Source: CAD feature listing. Evaluate the final solid. Frame: model axes, mm. A direction names the side the tool comes from. Give positions to 0.01 mm unless a question says otherwise; leave off trailing zeros. Loops run counter-clockwise (first coordinate to the right, second up) from the corner with the lowest first, then second, coordinate; pieces in that order, holes last. Notation, with made-up numbers: (-39, -28.5) -> (-8, -28.5) arc R11 cw to (-8, -10.5) -> close; hole circle Ø3 at (53.5, 29.25). An arc over 180 degrees is marked (long way). Return JSON: item names as keys, results as strings. Group by question number.
```python
from build123d import *

# Parameters (mm, degrees)
BOSS_EXTRUDE1_DEPTH = 1.3
SKETCH2_W           = 1.4
SKETCH2_H           = 18
BOSS_EXTRUDE2_DEPTH = 1.3
SKETCH2_3_W         = 25
SKETCH2_3_H         = 16
CUT_EXTRUDE1_DEPTH  = 55.166871794
CUT_EXTRUDE2_DEPTH  = 55.166871794
SKETCH7_W           = 1
SKETCH7_H           = 14
CUT_EXTRUDE3_DEPTH  = 55.166871794


with BuildPart() as part:
    # Sketch1 → Boss-Extrude1 (new body)
    with BuildSketch(Plane(origin=(0, 0, 0), x_dir=(1, 0, 0), z_dir=(0, 1, 0))):
        Polygon((-43, 31), (43, 31), (43, -20), (32, -31), (-32, -31), (-43, -20), align=None)
    extrude(amount=BOSS_EXTRUDE1_DEPTH)

    # Sketch2 → Boss-Extrude2 (add)
    with BuildSketch(Plane(origin=(0, 0, 0), x_dir=(1, 0, 0), z_dir=(0, 1, 0))):
        with Locations((43.7, 2)):
            Rectangle(SKETCH2_W, SKETCH2_H)
        with Locations((-43.7, 2)):
            Rectangle(SKETCH2_W, SKETCH2_H)
    extrude(amount=BOSS_EXTRUDE2_DEPTH)

    # Sketch2<3> → Cut-Extrude1 (cut, through all)
    with BuildSketch(Plane(origin=(0, 0, 0), x_dir=(1, 0, 0), z_dir=(0, 1, 0))):
        with Locations((0, 23)):
            Rectangle(SKETCH2_3_W, SKETCH2_3_H)
    extrude(amount=CUT_EXTRUDE1_DEPTH, mode=Mode.SUBTRACT)

    # Sketch6 → Cut-Extrude2 (cut, through all)
    with BuildSketch(Plane(origin=(0, 1.3, 0), x_dir=(1, 0, 0), z_dir=(0, 1, 0))):
        with BuildLine():
            Line((-43, 31), (43, 31))
            ThreePointArc((43, 31), (0, 23.231359566), (-43, 31))
        make_face()
    extrude(amount=-CUT_EXTRUDE2_DEPTH, mode=Mode.SUBTRACT)

    # Sketch7 → Cut-Extrude3 (cut, through all)
    with BuildSketch(Plane(origin=(0, 1.3, 0), x_dir=(1, 0, 0), z_dir=(0, 1, 0))):
        with Locations((-10.5, -5.25)):
            Rectangle(SKETCH7_W, SKETCH7_H)
        with Locations((10.5, -5.25)):
            Rectangle(SKETCH7_W, SKETCH7_H)
    extrude(amount=-CUT_EXTRUDE3_DEPTH, mode=Mode.SUBTRACT)


solid = part.part
```
1) Reachability of faces 1 (the face through (1, 1.3, 0)), 2 (the face through (-27.764, 0.659, -26.409)) from +Z, -Z, +X, -X, +Y, -Y: full face, straight path, thin tool, end or side. Return the list, or none.
2) Mould query, pull axis X, two halves, no side actions, for faces 3 (the face through (28.19, 0.66, -26.51)), 4 (the face through (1, 0, 0)), 5 (the face through (38, 1, 25)). Classes: released by +X, released by -X, zero draft, split by the parting line, or undercut.
3) Material intervals for line 1 (X direction, y = 0.5, z = 8.5); line 2 (X direction, y = 0.6, z = 3); line 3 (X direction, y = 0.1, z = 17.5), sorted ascending.
4) Cut plane C-C on z = -21. Return loops of the section in (x, y).
5) Cut plane A-A on z = 8. Return loops of the section in (x, y).
6) Contact query for flat-ended pins moving along their axis: P1, Ø0.6, axis at x = 44, y = 1, coming from the -Z side; P2, Ø0.6, axis at y = 0.5, z = -18.5, coming from the -X side; P3, Ø0.6, axis at y = 1, z = -20.5, coming from the +X side. Output: stop coordinate, or through.
7) Cut plane B-B on y = 1.05. Return loops of the section in (x, z), then the cut area to 3 significant figures.
8) Cut plane D-D on x = -2. Return loops of the section in (y, z).
Calculated:
{
 "1": {"face 1": "+Z, -Z, +X, -X, +Y", "face 2": "-Z, +Y, -Y"},
 "2": {"face 3": "undercut", "face 4": "zero draft", "face 5": "released by +X"},
 "3": {"line 1": "-43 to -11, -10 to 10, 11 to 43", "line 2": "-44.4 to -11, -10 to 10, 11 to 44.4", "line 3": "-43 to 43"},
 "4": {"outline": "(-43, 0) -> (-12.5, 0) -> (-12.5, 1.3) -> (-43, 1.3) -> close; (12.5, 0) -> (43, 0) -> (43, 1.3) -> (12.5, 1.3) -> close"},
 "5": {"outline": "(-43, 0) -> (-11, 0) -> (-11, 1.3) -> (-43, 1.3) -> close; (-10, 0) -> (10, 0) -> (10, 1.3) -> (-10, 1.3) -> close; (11, 0) -> (43, 0) -> (43, 1.3) -> (11, 1.3) -> close"},
 "6": {"P1": "z = -11", "P2": "x = -43", "P3": "x = 43"},
 "7": {"outline": "(-44.4, -11) -> (-43, -11) -> (-43, -31) arc R122.89 cw to (-12.5, -23.87) -> (-12.5, -15) -> (12.5, -15) -> (12.5, -23.87) arc R122.89 cw to (43, -31) -> (43, -11) -> (44.4, -11) -> (44.4, 7) -> (43, 7) -> (43, 20) -> (32, 31) -> (-32, 31) -> (-43, 20) -> (-43, 7) -> (-44.4, 7) -> close; hole (-11, -1.75) -> (-10, -1.75) -> (-10, 12.25) -> (-11, 12.25) -> close; hole (10, -1.75) -> (11, -1.75) -> (11, 12.25) -> (10, 12.25) -> close", "area": "4,570 mm2"},
 "8": {"outline": "(0, -15) -> (1.3, -15) -> (1.3, 31) -> (0, 31) -> close"}
}
